from build123d import *

# Parameters (mm, degrees)
F0_R            = 80.749
F0_R_2          = 4.875
F0_R_3          = 20.6375
F1_DEPTH        = 20
F2_D            = 13.49248
F2_COPIES_COUNT = 5
F3_D            = 6.7564
F3_COPIES_COUNT = 10


# Not quite as in the source:
# - a pattern or mirror of a feature is missing from the dataset's text; its kind, count and spacing are read off the source's solid
# - a feature names something its author has since deleted; it is built from what else it names


with BuildPart() as f1:
    # F0 (on Front) → F1 (new body)
    with BuildSketch(Plane.XZ):
        Circle(F0_R)
        with Locations((-22.9412823532, -50.481680479)):
            Circle(F0_R_2, mode=Mode.SUBTRACT)
        with Locations((-40.9216850532, -37.4181532468)):
            Circle(F0_R_2, mode=Mode.SUBTRACT)
        Circle(F0_R_3, mode=Mode.SUBTRACT)
        with Locations((22.9412823532, -50.481680479)):
            Circle(F0_R_2, mode=Mode.SUBTRACT)
        with Locations((40.9216850532, -37.4181532468)):
            Circle(F0_R_2, mode=Mode.SUBTRACT)
        with Locations((-55.100177293, 6.2187589016)):
            Circle(F0_R_2, mode=Mode.SUBTRACT)
        with Locations((-48.2322745931, 27.3559899762)):
            Circle(F0_R_2, mode=Mode.SUBTRACT)
        with Locations((-11.1125, 54.3250848481)):
            Circle(F0_R_2, mode=Mode.SUBTRACT)
        with Locations((55.100177293, 6.2187589016)):
            Circle(F0_R_2, mode=Mode.SUBTRACT)
        with Locations((48.2322745931, 27.3559899762)):
            Circle(F0_R_2, mode=Mode.SUBTRACT)
        with Locations((11.1125, 54.3250848481)):
            Circle(F0_R_2, mode=Mode.SUBTRACT)
        with Locations((-55.100177293, 6.2187589016)):
            Circle(F0_R_2)
        with Locations((-40.9216850532, -37.4181532468)):
            Circle(F0_R_2)
        with Locations((-22.9412823532, -50.481680479)):
            Circle(F0_R_2)
        with Locations((55.100177293, 6.2187589016)):
            Circle(F0_R_2)
        with Locations((48.2322745931, 27.3559899762)):
            Circle(F0_R_2)
        with Locations((11.1125, 54.3250848481)):
            Circle(F0_R_2)
    extrude(amount=F1_DEPTH)

    # F2 (through all)
    with Locations(Plane(origin=(0, 0, 0), x_dir=(1, 0, 0), z_dir=(0, 1, 0))):
        with Locations((-26.4503363532, -36.4057647469)):
            f2 = Hole(F2_D / 2)

    # F2_copies: F2 ×5 about axis
    f2_copies_axis = Axis((0, 0, 0), (0, 1, 0))
    for i in range(1, F2_COPIES_COUNT):
        add(f2.rotate(f2_copies_axis, i * 360 / F2_COPIES_COUNT), mode=Mode.SUBTRACT)

    # F3 (through all)
    with Locations(Plane(origin=(0, 0, 0), x_dir=(1, 0, 0), z_dir=(0, 1, 0))):
        with Locations((-41.0567998726, -56.5098370571)):
            f3 = Hole(F3_D / 2)

    # F3_copies: F3 ×10 about axis
    f3_copies_axis = Axis((0, 0, 0), (0, 1, 0))
    for i in range(1, F3_COPIES_COUNT):
        add(f3.rotate(f3_copies_axis, i * 360 / F3_COPIES_COUNT), mode=Mode.SUBTRACT)


solid = f1.part
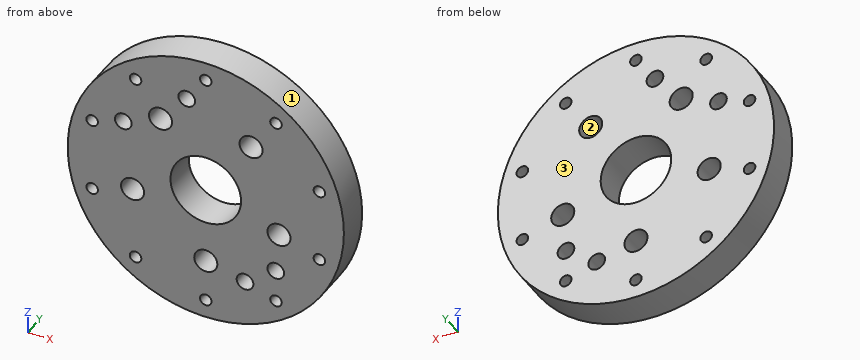
The listing builds one solid part. Answer for the finished solid, in the listing's coordinates (mm). Face numbers are marked on the shaded views. Give positions to 0.01 mm unless a question says otherwise; leave off trailing zeros. Order: outer loops, then holes, each group sorted by start corner. A loop starts at its lowest first (then second) coordinate and runs counter-clockwise, first axis right, second up. Notation, with made-up numbers: (39.5, 79.25) - (84.5, 79.25) arc R8 ccw to (84.5, 88.25) - close; hole circle Ø9 at (12.25, -9.5). An arc over 180 degrees is marked (long way). Answer as CSV lines item,"result".
Q1. A cutting plane is placed at A-A, the plane x = 0. Determine the outline of the cut face in (y, z).
Answer key:
outline,"(-20, -80.75) - (0, -80.75) - (0, -73.23) - (-20, -73.23) - close; (-20, -66.47) - (0, -66.47) - (0, -51.75) - (-20, -51.75) - close; (-20, -38.25) - (0, -38.25) - (0, -20.64) - (-20, -20.64) - close; (-20, 20.64) - (0, 20.64) - (0, 66.47) - (-20, 66.47) - close; (-20, 73.23) - (0, 73.23) - (0, 80.75) - (-20, 80.75) - close"
Q2. Each of these flat-tipped pins is pushed along its axis until it touches: pin 1 Ø12 at (y, z) = (-5, -31.5) entering from +X; pin 2 Ø12 at (y, z) = (-13.5, 22) entering from -X; pin 3 Ø2 at (x, y) = (35, -3.5) entering from +Z. Where does it stop, or does it pass through?
Answer key:
pin 1,"stops at x = 76.62"
pin 2,"stops at x = -79.15"
pin 3,"stops at z = 73.24"
Q3. A cutting plane is placed at D-D, the plane z = -15. Determine the outline of the cut face in (x, y), and give its area (3 significant figures).
Answer key:
outline,"(-79.34, -20) - (-49.45, -20) - (-49.45, 0) - (-79.34, 0) - close; (-36.14, -20) - (-14.17, -20) - (-14.17, 0) - (-36.14, 0) - close; (14.17, -20) - (36.14, -20) - (36.14, 0) - (14.17, 0) - close; (49.45, -20) - (79.34, -20) - (79.34, 0) - (49.45, 0) - close"
area,"2,070 mm^2"
Q4. A cutting plane is placed at B-B, the plane z = 2.5. Determine the outline of the cut face in (x, y).
Answer key:
outline,"(-80.71, -20) - (-20.49, -20) - (-20.49, 0) - (-80.71, 0) - close; (20.49, -20) - (80.71, -20) - (80.71, 0) - (20.49, 0) - close"
Q5. Straight lines are drawn through the part: L1, parallel to Z at x = 24, y = -11.75; L2, parallel to X at y = -16.5, z = -9; L3, parallel to X at y = -7.75, z = 37.5. For each, find the intervals that lie inside material, in ascending order.
Answer key:
L1,"z = -77.1 to -55.24, -45.72 to 30.12, 42.69 to 77.1"
L2,"x = -80.25 to -47.43, -38.17 to -18.57, 18.57 to 38.17, 47.43 to 80.25"
L3,"x = -71.51 to -33.11, -19.79 to 19.79, 33.11 to 71.51"
Q6. Determine the mould class of the marked faces 1, 2 and 3 for opening direction Z: pulls with the +Z half, pulls with the -Z half, needs draft (parallel to the pull), parting line crosses it, or undercut.
Answer key:
face 1,"parting line crosses it"
face 2,"undercut"
face 3,"needs draft"
Q7. A cutting plane is placed at C-C, the plane y = -2. Count the separate pieces of the cut face and the enclosed holes in it, and give its area (3 significant figures).
Answer key:
separate pieces,"1"
enclosed holes,"20"
area,"17,800 mm^2"
